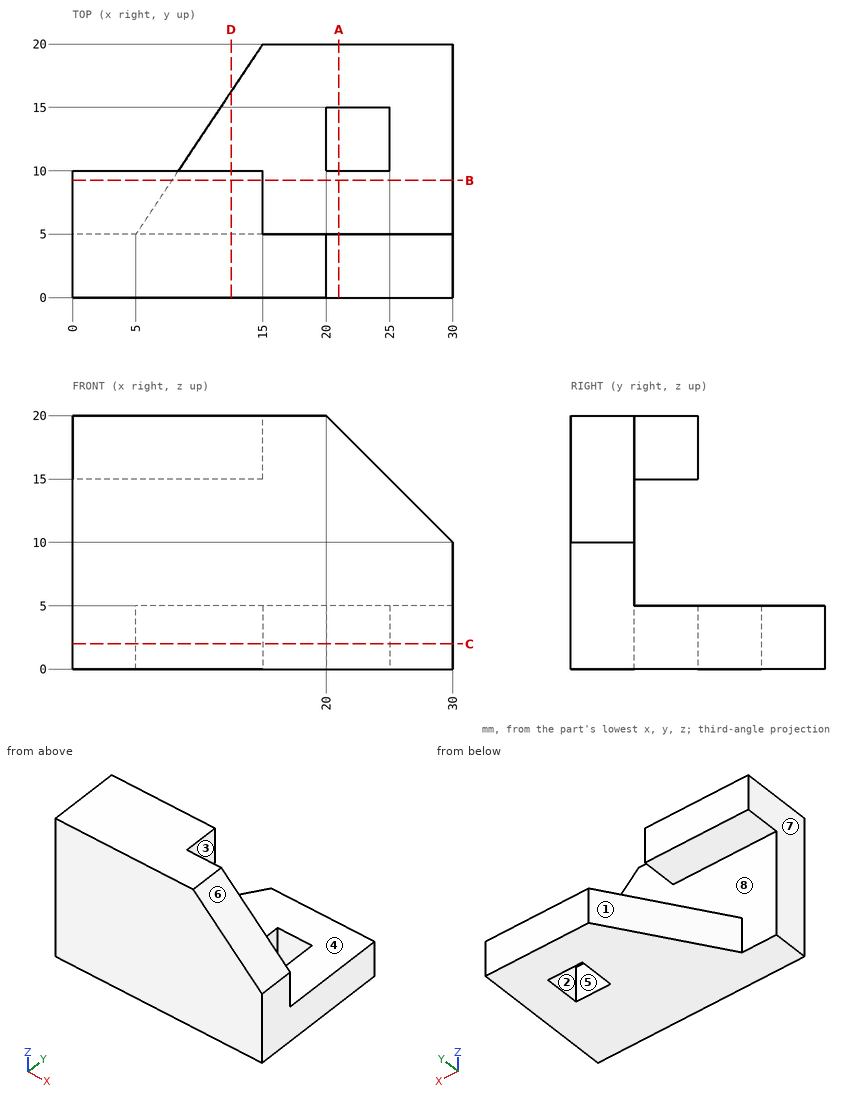
Geometry: see drawing. Coordinates: mm, zero at the bounding-box minimum. A direction names the side the tool comes from. Give positions to 0.01 mm unless a question says otherwise; leave off trailing zeros. Loops run counter-clockwise (first coordinate to the right, second up) from the corner with the lowest first, then second, coordinate; pieces in that order, holes last. Notation, with made-up numbers: (83.25, -5.75) -> (111.25, -5.75) arc R12 cw to (111.25, -0.75) -> close; hole circle Ø7 at (18, -23). An arc over 180 degrees is marked (long way). Use CSV: the item, a comma, the result in double quotes.
(1) Cut plane A-A (x = 21). Output: boundary loops of the cut face in (y, z).
From the geometry:
outline,"(0, 0) -> (10, 0) -> (10, 5) -> (5, 5) -> (5, 19) -> (0, 19) -> close; (15, 0) -> (20, 0) -> (20, 5) -> (15, 5) -> close"
(2) Cut plane B-B (y = 9.25). Output: boundary loops of the cut face in (x, z), plus the area to 3 significant figures.
From the geometry:
outline,"(0, 15) -> (15, 15) -> (15, 20) -> (0, 20) -> close; (7.83, 0) -> (30, 0) -> (30, 5) -> (7.83, 5) -> close"
area,"186 mm^2"
(3) Cut plane D-D (x = 12.5). Output: boundary loops of the cut face in (y, z), plus the area to 3 significant figures.
From the geometry:
outline,"(0, 0) -> (16.25, 0) -> (16.25, 5) -> (5, 5) -> (5, 15) -> (10, 15) -> (10, 20) -> (0, 20) -> close"
area,"181 mm^2"
(4) Access query for the marked faces 1, 2, 3 and 4. Directions: +Z, -Z, +X, -X, +Y, -Y. A direction counts if a zero-diameter tool reaches every point of the face in a straight line with its end or side. Return the directions, or none.
From the geometry:
face 1,"-Z, -X, +Y"
face 2,"+Z, -Z"
face 3,"+Z, +X, +Y"
face 4,"+X, -X, +Y"
(5) Cut plane C-C (z = 2). Output: boundary loops of the cut face in (x, y).
From the geometry:
outline,"(0, 0) -> (30, 0) -> (30, 20) -> (15, 20) -> (5, 5) -> (0, 5) -> close; hole (20, 10) -> (25, 10) -> (25, 15) -> (20, 15) -> close"
(6) Pull-direction query (X, two-part tool) for the marked faces 5, 6, 7 and 8; classes: released by +X, released by -X, zero draft, split by the parting line, or undercut.
From the geometry:
face 5,"undercut"
face 6,"released by +X"
face 7,"released by -X"
face 8,"zero draft"
(7) Ray query, line 1 along Z through (x, y) = (26.5, 6.5); line 2 along Z through (x, y) = (5, 7). Return the intervals inside material, ascending. Write a range as [from, to].
From the geometry:
line 1,"[0, 5]"
line 2,"[15, 20]"
(8) First-contact query: P1, Ø4, axis at y = 8, z = 18.5, coming from the +X side; P2, Ø1.5, axis at y = 12.5, z = 3.5, coming from the -X side; P3, Ø6, axis at x = 16, y = 15, coming from the +Z side; P4, Ø1.5, axis at y = 10.5, z = 13.5, coming from the -X side. Flat tips, straight axial feed; report the tip coordinate or a pass-through.
From the geometry:
P1,"x = 15"
P2,"x = 9.5"
P3,"z = 5"
P4,"through"
